from build123d import *

# Parameters (mm, degrees)
SKETCH_1_R      = 1
SKETCH_1_R_2    = 1.25
SKETCH_1_R_3    = 9.5
EXTRUDE_1_DEPTH = 2


with BuildPart() as part:
    # 草圖1 → 填料-伸長1 (new body)
    with BuildSketch(Plane.XY):
        with BuildLine():
            Line((-8.868434636, 14.893709246), (-8.868434636, 15.893709246))
            Line((-8.868434636, 15.893709246), (-7.868434636, 15.893709246))
            Line((-7.868434636, 15.893709246), (43.781565364, 15.893709246))
            Line((43.781565364, 15.893709246), (44.731565364, 15.893709246))
            Line((44.731565364, 15.893709246), (44.731565364, 14.893709246))
            Line((44.731565364, 14.893709246), (44.731565364, -15.106290754))
            Line((44.731565364, -15.106290754), (44.731565364, -16.106290754))
            Line((44.731565364, -16.106290754), (43.781565364, -16.106290754))
            Line((43.781565364, -16.106290754), (-7.868434636, -16.106290754))
            Line((-7.868434636, -16.106290754), (-8.868434636, -16.106290754))
            Line((-8.868434636, -16.106290754), (-8.868434636, -15.106290754))
            Line((-8.868434636, -15.106290754), (-8.868434636, -10.106290754))
            ThreePointArc((-8.868434636, -10.106290754), (-7.868434636, -9.106290754), (-8.868434636, -8.106290754))
            Line((-8.868434636, -8.106290754), (-10.868434636, -8.106290754))
            Line((-10.868434636, -8.106290754), (-10.868434636, -4.106290754))
            Line((-10.868434636, -4.106290754), (-8.868434636, -4.106290754))
            ThreePointArc((-8.868434636, -4.106290754), (-7.868434636, -3.106290754), (-8.868434636, -2.106290754))
            Line((-8.868434636, -2.106290754), (-8.868434636, 1.893709246))
            ThreePointArc((-8.868434636, 1.893709246), (-7.868434636, 2.893709246), (-8.868434636, 3.893709246))
            Line((-8.868434636, 3.893709246), (-10.868434636, 3.893709246))
            Line((-10.868434636, 3.893709246), (-10.868434636, 7.893709246))
            Line((-10.868434636, 7.893709246), (-8.868434636, 7.893709246))
            ThreePointArc((-8.868434636, 7.893709246), (-7.868434636, 8.893709246), (-8.868434636, 9.893709246))
            Line((-8.868434636, 9.893709246), (-8.868434636, 14.893709246))
        make_face()
        with Locations((-6.868434636, 5.893709246)):
            Circle(SKETCH_1_R, mode=Mode.SUBTRACT)
        with Locations((-6.868434636, -6.106290754)):
            Circle(SKETCH_1_R, mode=Mode.SUBTRACT)
        with Locations((-2.368434636, 13.393709246)):
            Circle(SKETCH_1_R_2, mode=Mode.SUBTRACT)
        with Locations((-2.368434636, -13.606290754)):
            Circle(SKETCH_1_R_2, mode=Mode.SUBTRACT)
        with Locations((27.631565364, 13.393709246)):
            Circle(SKETCH_1_R_2, mode=Mode.SUBTRACT)
        with Locations((27.631565364, -13.606290754)):
            Circle(SKETCH_1_R_2, mode=Mode.SUBTRACT)
        with Locations((29.131565364, -0.106290754)):
            Circle(SKETCH_1_R_3, mode=Mode.SUBTRACT)
    extrude(amount=EXTRUDE_1_DEPTH)


solid = part.part
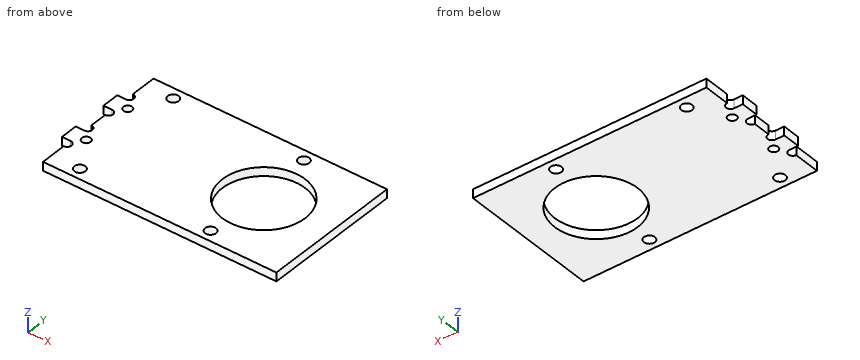
Verification items for the finished model (mm, model axes). Coordinates: 2 decimals unless noted, no trailing zeros. Order: outer loops, then holes, each group sorted by start corner. A loop starts at its lowest first (then second) coordinate and runs counter-clockwise, first axis right, second up. Notation, with made-up numbers: (20.25, 65) -> (65.25, 65) arc R22 cw to (65.25, 104) -> close; hole circle Ø4 at (80.25, 62.5). An arc over 180 degrees is marked (long way). Put each result on its own line as item: value. Start each with the question number.
1. Cross-section at C-C, the plane z = 1.25. Record the boundary of the cut face in (x, y).
2. Cross-section at B-B, the plane y = -1.5. Record the boundary of the cut face in (x, z), then the cut area to 3 significant figures.
3. Material ranges on L1, parallel to X at y = 13.5, z = 0.75; L2, parallel to X at y = -5.5, z = 1.6; L3, parallel to X at y = -2.5, z = 1.1, recorded low to high. Write a range as [from, to].
4. Go/stop test with flat-tipped pins: pin 1 Ø1 at (x, z) = (-9.5, 1) entering from -Y; pin 2 Ø1 at (y, z) = (-12, 1) entering from -X. Record where each tip stops, or that it passes through.
5. Cross-section at A-A, the plane x = 36.5. Record the boundary of the cut face in (y, z), then the cut area to 3 significant figures.
Computed:
1. outline: (-10.87, -8.11) -> (-8.87, -8.11) arc R1 cw to (-8.87, -10.11) -> (-8.87, -16.11) -> (44.73, -16.11) -> (44.73, 15.89) -> (-8.87, 15.89) -> (-8.87, 9.89) arc R1 cw to (-8.87, 7.89) -> (-10.87, 7.89) -> (-10.87, 3.89) -> (-8.87, 3.89) arc R1 cw to (-8.87, 1.89) -> (-8.87, -2.11) arc R1 cw to (-8.87, -4.11) -> (-10.87, -4.11) -> close; hole circle Ø2 at (-6.87, -6.11); hole circle Ø2 at (-6.87, 5.89); hole circle Ø2.5 at (-2.37, -13.61); hole circle Ø2.5 at (-2.37, 13.39); hole circle Ø19 at (29.13, -0.11); hole circle Ø2.5 at (27.63, -13.61); hole circle Ø2.5 at (27.63, 13.39)
2. outline: (-8.87, 0) -> (19.73, 0) -> (19.73, 2) -> (-8.87, 2) -> close; (38.53, 0) -> (44.73, 0) -> (44.73, 2) -> (38.53, 2) -> close
2. area: 69.6 mm2
3. L1: [-8.87, -3.61], [-1.12, 26.39], [28.88, 44.73]
3. L2: [-10.87, -7.66], [-6.07, 21.31], [36.95, 44.73]
3. L3: [-8.07, 19.94], [38.33, 44.73]
4. pin 1: y = -8.11
4. pin 2: x = -8.87
5. outline: (-16.11, 0) -> (-6.1, 0) -> (-6.1, 2) -> (-16.11, 2) -> close; (5.89, 0) -> (15.89, 0) -> (15.89, 2) -> (5.89, 2) -> close
5. area: 40.0 mm2
